Can you work these out from the model? Positions are in its coordinate system, mm. A direction names the side the tool comes from. Give positions to 0.01 mm unless a question says otherwise; leave off trailing zeros. Order: outer loops, then holes, each group sorted by start corner. A loop starts at its lowest first (then second) coordinate and runs counter-clockwise, first axis right, second up. Notation, with made-up numbers: (-27, 30.25) - (8, 30.25) arc R15 ccw to (8, 37.25) - close; hole circle Ø10 at (-13.5, 23). An arc over 180 degrees is marked (long way). One line per question, with ' | ' between items.
```python
from build123d import *

# Parameters (mm, degrees)
BOSS_EXTRUDE1_DEPTH = 16
SKETCH2_R           = 1.75
CUT_EXTRUDE1_DEPTH  = 8
SKETCH3_R           = 1.5
BOSS_EXTRUDE2_DEPTH = 5
CHAMFER1_SIZE       = 0.5


with BuildPart() as part:
    # Sketch1 → Boss-Extrude1 (new body)
    with BuildSketch(Plane.XY):
        Polygon((0, 2.75), (-2.38156986, 1.375), (-2.38156986, -1.375), (0, -2.75), (2.38156986, -1.375), (2.38156986, 1.375), align=None)
    extrude(amount=BOSS_EXTRUDE1_DEPTH)

    # Sketch2 → Cut-Extrude1 (cut)
    with BuildSketch(Plane.XY.offset(16)):
        Circle(SKETCH2_R)
    extrude(amount=-CUT_EXTRUDE1_DEPTH, mode=Mode.SUBTRACT)

    # Sketch3 → Boss-Extrude2 (add)
    with BuildSketch(Plane(origin=(0, 0, 0), x_dir=(-1, 0, 0), z_dir=(0, 0, -1))):
        with Locations(Location((0, 0, 0), (0, 0, 180))):
            Circle(SKETCH3_R)
    extrude(amount=BOSS_EXTRUDE2_DEPTH)

    # Chamfer1
    chamfer1_edges = [part.edges().sort_by_distance(p)[0] for p in [
        (-1.5, 0, -5),
    ]]
    chamfer(chamfer1_edges, length=CHAMFER1_SIZE)


solid = part.part
```
(1) Imagine slicing it at A-A (y = 0). List the corners of the cut face in (x, z) for me.
Answer below:
outline: (-2.38, 0) - (-1.5, 0) - (-1.5, -4.5) - (-1, -5) - (1, -5) - (1.5, -4.5) - (1.5, 0) - (2.38, 0) - (2.38, 16) - (1.75, 16) - (1.75, 8) - (-1.75, 8) - (-1.75, 16) - (-2.38, 16) - close
(2) Imagine slicing it at B-B (z = -1.5). List the corners of the cut face in (x, y) for me.
Answer below:
outline: circle Ø3 at (0, 0)
(3) On a 3-axis mill with a long thin cutter (end or side, diameter ignored), from which of +Z, -Z, +X, -X, +Y, -Y can I reach the whole of each face in a straight line? I mean faces 4 (the face through (2, 0, 0)), 5 (the face through (0, 0, 8)), 6 (the face through (1.21, 2.05, 7.89)). Say none if no direction works.
Answer below:
face 4: -Z | face 5: +Z | face 6: +Z, -Z, +X, +Y
(4) If we mould it in two halves opening along Y, with no side actions, what happens to faces 1 (the face through (1.617, -0.67, 12.056)), 2 (the face through (2.382, 0, 8)), 3 (the face through (1.174, -2.072, 7.888))? For each: released by +Y, released by -Y, zero draft, split by the parting line, or undercut.
Answer below:
face 1: undercut | face 2: zero draft | face 3: released by -Y
(5) Will these pins go through, and if not, where does the flat tip stop? pin 1 (2 mm diameter, centred on x = 0.5, z = 7, fed in from +Y); pin 2 (1.5 mm diameter, centred on x = 1.5, z = 1, fed in from -Y); pin 3 (2 mm diameter, centred on x = 1.5, z = -0.5, fed in from -Y).
Answer below:
pin 1: y = 2.75 | pin 2: y = -2.32 | pin 3: y = -2.38
(6) If I drill on line 1 (Z direction, x = 1.85, y = -1.15); line 2 (Z direction, x = -0.3, y = -0.15); line 3 (Y direction, x = -0.6, z = -1.5), over which ranges is the centre line in solid material (lowest first)?
Answer below:
line 1: 0 to 16 | line 2: -5 to 8 | line 3: -1.37 to 1.37
